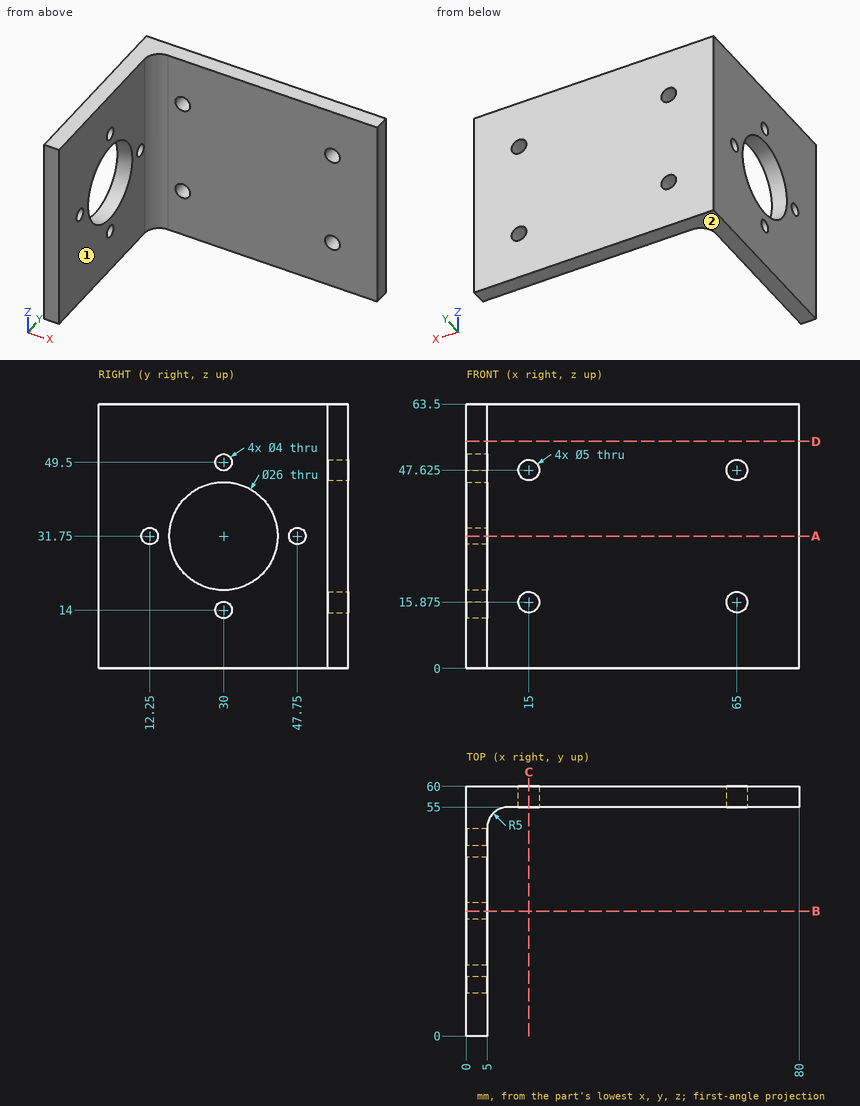
Geometry check sheet. Reference: drawing and pictorial views, mm from the part's lowest x, y, z. A direction names the side the tool comes from. Give positions to 0.01 mm unless a question says otherwise; leave off trailing zeros. Write each loop counter-clockwise with the first axis right and the second up, starting at its lowest first coordinate (ties: lowest second). Pieces come first, ordered by that corner, then holes. Notation, with made-up numbers: (-17.75, -2.5) - (3.25, -2.5) arc R17 cw to (3.25, 28.5) - close; hole circle Ø5 at (-21, -34.5). An arc over 180 degrees is marked (long way). Use a Markdown table: item, result.
Q1. Go/stop test with flat-tipped pins: P1, Ø3, axis at x = 33, z = 22.5, coming from the -Y side; P2, Ø12, axis at x = 12, z = 13.5, coming from the -Y side; P3, Ø25, axis at y = 35.5, z = 30.5, coming from the +X side. Record where each tip stops, or that it passes through.
Computed:
| item | result |
|---|---|
| P1 | stops at y = 55 |
| P2 | stops at y = 53 |
| P3 | stops at x = 5 |
Q2. Section check C-C, the plane x = 15. Enter the section's corners in (y, z) (3 decimals), then the cut area to 4 significant figures.
Computed:
| item | result |
|---|---|
| outline | (55, 0) - (60, 0) - (60, 13.375) - (55, 13.375) - close; (55, 18.375) - (60, 18.375) - (60, 45.125) - (55, 45.125) - close; (55, 50.125) - (60, 50.125) - (60, 63.5) - (55, 63.5) - close |
| area | 267.5 mm² |
Q3. Section check A-A, the plane z = 31.75. Enter the section's corners in (x, y), then the cut area to 3 significant figures.
Computed:
| item | result |
|---|---|
| outline | (0, 0) - (5, 0) - (5, 10.25) - (0, 10.25) - close; (0, 14.25) - (5, 14.25) - (5, 17) - (0, 17) - close; (0, 43) - (5, 43) - (5, 45.75) - (0, 45.75) - close; (0, 49.75) - (5, 49.75) - (5, 50) arc R5 cw to (10, 55) - (80, 55) - (80, 60) - (0, 60) - close |
| area | 510 mm² |
Q4. Section check B-B, the plane y = 30. Enter the section's corners in (x, z), then the cut area to 4 significant figures.
Computed:
| item | result |
|---|---|
| outline | (0, 0) - (5, 0) - (5, 12) - (0, 12) - close; (0, 16) - (5, 16) - (5, 18.75) - (0, 18.75) - close; (0, 44.75) - (5, 44.75) - (5, 47.5) - (0, 47.5) - close; (0, 51.5) - (5, 51.5) - (5, 63.5) - (0, 63.5) - close |
| area | 147.5 mm² |
Q5. Set-up check for the marked faces 1 and 2: record each of +Z, -Z, +X, -X, +Y, -Y from which the full face is reachable in a straight line by a thin tool's end or side.
Computed:
| item | result |
|---|---|
| face 1 | +Z, -Z, +X, -Y |
| face 2 | -Z, +X, -X, +Y, -Y |
Q6. Thickness scan on L1, parallel to Z at x = 15, y = 59.05 (3 decimals); L2, parallel to Y at x = 3.5, z = 31.75; L3, parallel to Y at x = 1.15, z = 49.5. Record the ranges inside material, lowest first. Write a range as [from, to].
Computed:
| item | result |
|---|---|
| L1 | z = [0, 13.375], [18.375, 45.125], [50.125, 63.5] |
| L2 | y = [0, 10.25], [14.25, 17], [43, 45.75], [49.75, 60] |
| L3 | y = [0, 28], [32, 60] |
Q7. Section check D-D, the plane z = 54.5. Enter the section's corners in (x, y).
Computed:
| item | result |
|---|---|
| outline | (0, 0) - (5, 0) - (5, 50) arc R5 cw to (10, 55) - (80, 55) - (80, 60) - (0, 60) - close |
